Can you work these out from the model? Positions are in its coordinate system, mm. A direction names the side the tool comes from. Coordinates: 2 decimals unless noted, no trailing zeros. Order: outer loops, then holes, each group sorted by start corner. A loop starts at its lowest first (then second) coordinate and runs counter-clockwise, first axis right, second up. Notation, with made-up numbers: (1.5, 39) -> (54.5, 39) arc R12 ccw to (54.5, 51) -> close; hole circle Ø3 at (-1.75, -11.75). An arc over 180 degrees is marked (long way). Answer as a JSON object with one key per item and string values. Group by question number.
(1) I want a section at D-D, the plane z = -4. List the corners of the cut face in (x, y) for me (3 decimals).
(2) For pin 1 (1.3 mm diameter, centred on y = -8, z = 1, fed in from +X); pin 2 (1 mm diameter, centred on x = 7, y = 6, fed in from +Z); pin 3 (2 mm diameter, centred on x = 10.5, z = -1.5, fed in from -Y) (3 decimals), each with a flat end and sliding along its axis, tell me the tip position at first contact or that it passes through.
(3) Which directions (+Z, -Z, +X, -X, +Y, -Y) give clear straight access to the entire face, cutting with the end or side of a thin tool? Please do faces 1 (the flat face through (6.35, -8, 0)), 2 (the cylindrical face through (2.962, -0.866, 1.295)).
(4) I need wall thicknesses on line 1 (Y direction, x = 3.55, z = 0) (3 decimals); line 2 (X direction, y = -6, z = 4); line 3 (Y direction, x = 8, z = -3.5) (3 decimals). Which ranges of each line are inside material? Lowest first, please.
(5) If we mould it in two halves opening along Y, with no side actions, what happens to faces 3 (the flat face through (6, 9.525, 0)), 4 (the flat face through (5.842, -2, 0)), 5 (the flat face through (3, 0, -6.35))? For each: pulls with the +Y half, pulls with the -Y half, needs draft (parallel to the pull), parting line crosses it, or undercut.
(6) I want a section at C-C, the plane x = 7. List the corners of the cut face in (y, z) for me (3 decimals).
(7) I want a section at B-B, the plane y = -0.5. List the corners of the cut face in (x, z) for me, plus the area to 3 significant figures.
(8) I want a section at A-A, the plane z = 0. List the corners of the cut face in (x, y) for me (3 decimals).
from build123d import *

# Parameters (mm, degrees)
SKETCH1_W             = 12.7
SKETCH1_H             = 19.05
BOSS_EXTRUDE1_DEPTH   = 12.7
SKETCH2_W             = 6.35
SKETCH2_H             = 16.51
CUT_EXTRUDE1_DEPTH    = 21.329919454
SKETCH3_W             = 0.508
SKETCH3_H             = 13.97
CUT_EXTRUDE2_DEPTH    = 21.329919454
F_4_CLEARANCE_HOLE1_D = 3.2639


with BuildPart() as part:
    # Sketch1 → Boss-Extrude1 (new body)
    with BuildSketch(Plane(origin=(0, 0, 0), x_dir=(0, 0, -1), z_dir=(1, 0, 0))):
        Rectangle(SKETCH1_W, SKETCH1_H)
    extrude(amount=BOSS_EXTRUDE1_DEPTH)

    # Sketch2 → Cut-Extrude1 (cut, through all)
    with BuildSketch(Plane.XY.offset(6.35)):
        with Locations((9.525, -1.27)):
            Rectangle(SKETCH2_W, SKETCH2_H)
    extrude(amount=-CUT_EXTRUDE1_DEPTH, mode=Mode.SUBTRACT)

    # Sketch3 → Cut-Extrude2 (cut, through all)
    with BuildSketch(Plane.XY.offset(6.35)):
        with Locations((6.096, 0)):
            Rectangle(SKETCH3_W, SKETCH3_H)
    extrude(amount=-CUT_EXTRUDE2_DEPTH, mode=Mode.SUBTRACT)

    # #4 Clearance Hole1 (through all)
    with Locations(Plane.ZY):
        with Locations((0, 0.127)):
            Hole(F_4_CLEARANCE_HOLE1_D / 2)


solid = part.part
Computed values:
{
 "1": {"outline": "(0, -9.525) -> (6.35, -9.525) -> (6.35, -6.985) -> (5.842, -6.985) -> (5.842, 6.985) -> (12.7, 6.985) -> (12.7, 9.525) -> (0, 9.525) -> close"},
 "2": {"pin 1": "stops at x = 6.35", "pin 2": "passes through", "pin 3": "stops at y = 6.985"},
 "3": {"face 1": "+Z, -Z, +X, -Y", "face 2": "+X, -X"},
 "4": {"line 1": "y = -9.525 to -1.505, 1.759 to 9.525", "line 2": "x = 0 to 5.84", "line 3": "y = 6.985 to 9.525"},
 "5": {"face 3": "pulls with the +Y half", "face 4": "undercut", "face 5": "needs draft"},
 "6": {"outline": "(6.985, -6.35) -> (9.525, -6.35) -> (9.525, 6.35) -> (6.985, 6.35) -> close"},
 "7": {"outline": "(0, -6.35) -> (5.84, -6.35) -> (5.84, -1.51) -> (0, -1.51) -> close; (0, 1.51) -> (5.84, 1.51) -> (5.84, 6.35) -> (0, 6.35) -> close", "area": "56.6 mm2"},
 "8": {"outline": "(0, -9.525) -> (6.35, -9.525) -> (6.35, -6.985) -> (5.842, -6.985) -> (5.842, -1.505) -> (0, -1.505) -> close; (0, 1.759) -> (5.842, 1.759) -> (5.842, 6.985) -> (12.7, 6.985) -> (12.7, 9.525) -> (0, 9.525) -> close"}
}
